from build123d import *

# Parameters (mm, degrees)
F0_R     = 9.525
F0_W     = 19.05
F0_H     = 2.596250779
F1_DEPTH = 7.62
F2_DEPTH = 76.2
F3_R     = 3.81
F4_DEPTH = 25.4
F3_W     = 19.05
F3_H     = 11.43
F5_DEPTH = 2.54


with BuildPart() as f1:
    # F0 (on Top) → F1 (new body)
    with BuildSketch(Plane.XY):
        with BuildLine():
            Line((9.525, 24.2291148752), (9.525, 30.287569645))
            ThreePointArc((9.525, 30.287569645), (0, 31.75), (-9.525, 30.287569645))
            Line((-9.525, 30.287569645), (-9.525, 24.2291148752))
            Line((-9.525, 24.2291148752), (9.525, 24.2291148752))
        make_face()
        with BuildLine():
            ThreePointArc((-9.525, 30.287569645), (-18.7835533113, -25.5976683508), (31.75, 0))
            ThreePointArc((31.75, 0), (25.5976683508, 18.7835533113), (9.525, 30.287569645))
            Line((9.525, 30.287569645), (9.525, 24.2291148752))
            Line((9.525, 24.2291148752), (9.525, 21.6328640962))
            Line((9.525, 21.6328640962), (-9.525, 21.6328640962))
            Line((-9.525, 21.6328640962), (-9.525, 24.2291148752))
            Line((-9.525, 24.2291148752), (-9.525, 30.287569645))
        make_face()
        Circle(F0_R, mode=Mode.SUBTRACT)
        with Locations((0, 22.9309894857)):
            Rectangle(F0_W, F0_H)
    extrude(amount=F1_DEPTH)

    # F0 (on Top) → F2 (join)
    with BuildSketch(Plane.XY):
        with BuildLine():
            Line((9.525, 24.2291148752), (9.525, 30.287569645))
            ThreePointArc((9.525, 30.287569645), (0, 31.75), (-9.525, 30.287569645))
            Line((-9.525, 30.287569645), (-9.525, 24.2291148752))
            Line((-9.525, 24.2291148752), (9.525, 24.2291148752))
        make_face()
    extrude(amount=F2_DEPTH)

    # F3 (on face) → F4 (cut)
    with BuildSketch(Plane.XZ.offset(-24.2291148752)):
        with Locations((0, 66.04)):
            Circle(F3_R)
    extrude(amount=-F4_DEPTH, mode=Mode.SUBTRACT)

    # F3 (on face) → F5 (cut)
    with BuildSketch(Plane.XZ.offset(-24.2291148752)):
        with Locations((0, 66.04)):
            Rectangle(F3_W, F3_H)
        with Locations((0, 66.04)):
            Circle(F3_R, mode=Mode.SUBTRACT)
    extrude(amount=-F5_DEPTH, mode=Mode.SUBTRACT)


solid = f1.part
Read the model definition and answer for the solid it produces. Units are mm, in the model's axes. A direction names the side the tool comes from. Give positions to 0.01 mm unless a question says otherwise; leave off trailing zeros. Write each loop counter-clockwise with the first axis right and the second up, starting at its lowest first coordinate (ties: lowest second). Pieces come first, ordered by that corner, then holes. Notation, with made-up numbers: (43.25, 1.5) - (73.25, 1.5) arc R14 ccw to (73.25, 19.5) - close; hole circle Ø5 at (54.5, -32). An arc over 180 degrees is marked (long way). Use CSV: the item, a comma, the result in double quotes. Start each with the question number.
(1) Find section C-C (z = 66.04). Give the vertices of the cut face in (x, y) (3 decimals).
(2) Find section B-B (y = -4). Give the vertices of the cut face in (x, z), plus the area to 3 significant figures.
(3) Find section D-D (z = 57). Give the vertices of the cut face in (x, y) (3 decimals).
(4) Find section A-A (x = 0). Give the vertices of the cut face in (y, z) (3 decimals), plus the area to 3 significant figures.
(5) Consider line 1 along Z through (x, y) = (0, 30.55); line 2 along Y through (x, z) = (0, 1.5) (3 decimals); line 3 along X through (y, z) = (28.8, 66.04) (3 decimals). Determine where each line is inside the solid, lowest interval first.
(6) Given P1, Ø6.5, axis at y = 28, z = 49.5, coming from the -X side (3 decimals); P2, Ø21, axis at x = 3.5, z = 24.5, coming from the -Y side; P3, Ø5.5, axis at x = 0.5, z = 68, coming from the -Y side, each flat-ended and moving along its own axis, determine where each tip first touches the part or whether it passes through.
(7) For faces 1 (the flat face through (0, 24.229, 74)), 2 (the flat face through (0, 25, 60.325)), 3 (the flat face through (9.525, 27, 41)), 4 (the cylindrical face through (-7.559, -5.796, 3.757)), determine the directions among +Z, -Z, +X, -X, +Y, -Y from which every point of the face is accessible in a straight line to the end or side of a thin tool.
(8) Determine the mould class of faces 5 (the flat face through (0, 25, 71.755)), 6 (the flat face through (7, 8, 0)), 7 (the flat face through (-9.525, 27, 41)) for opening direction Z: +Z half, -Z half, draft (parallel to the pull), parting line (faces both ways), or undercut.
Findings below:
1,outline,"(-9.525, 26.769) - (-3.81, 26.769) - (-3.81, 31.521) arc R31.75 ccw to (-9.525, 30.288) - close; (3.81, 26.769) - (9.525, 26.769) - (9.525, 30.288) arc R31.75 ccw to (3.81, 31.521) - close"
2,outline,"(-31.5, 0) - (-8.64, 0) - (-8.64, 7.62) - (-31.5, 7.62) - close; (8.64, 0) - (31.5, 0) - (31.5, 7.62) - (8.64, 7.62) - close"
2,area,"348 mm2"
3,outline,"(-9.525, 24.229) - (9.525, 24.229) - (9.525, 30.288) arc R31.75 ccw to (-9.525, 30.288) - close"
4,outline,"(-31.75, 0) - (-9.525, 0) - (-9.525, 7.62) - (-31.75, 7.62) - close; (9.525, 0) - (31.75, 0) - (31.75, 62.23) - (26.769, 62.23) - (26.769, 60.325) - (24.229, 60.325) - (24.229, 7.62) - (9.525, 7.62) - close; (24.229, 71.755) - (26.769, 71.755) - (26.769, 69.85) - (31.75, 69.85) - (31.75, 76.2) - (24.229, 76.2) - close"
4,area,"788 mm2"
5,line 1,"0 to 62.23, 69.85 to 76.2"
5,line 2,"-31.75 to -9.525, 9.525 to 31.75"
5,line 3,"-9.525 to -3.81, 3.81 to 9.525"
6,P1,"x = -9.525"
6,P2,"y = 24.23"
6,P3,"y = 26.77"
7,face 1,"+Z, +X, -X, -Y"
7,face 2,"+X, -X, -Y"
7,face 3,"+Z, +X, +Y, -Y"
7,face 4,"+Z, -Z"
8,face 5,"undercut"
8,face 6,"-Z half"
8,face 7,"draft"
